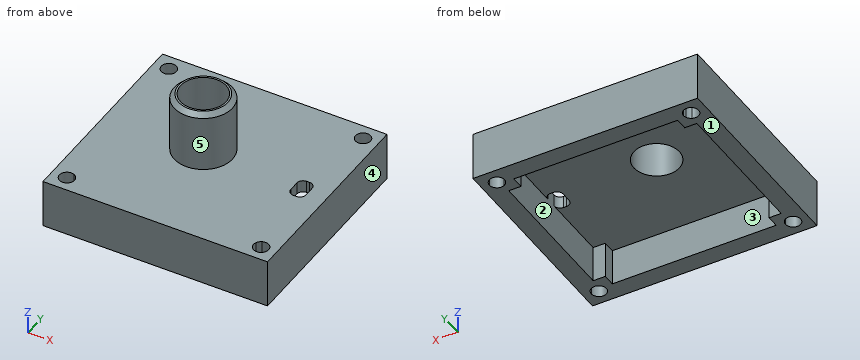
from build123d import *

# Parameters (mm, degrees)
F0_W     = 37
F0_H     = 34
F1_DEPTH = 8
F2_START = 6
F0_R     = 4.8
F2_DEPTH = 2
F3_R     = 1
F4_START = 6
F0_R_2   = 3.75
F4_DEPTH = 12
F5_SIZE  = 0.75


with BuildPart() as f1:
    # F0 (on Top) → F1 (new body)
    with BuildSketch(Plane.XY):
        with Locations((2.5, -1)):
            Rectangle(F0_W, F0_H)
        with BuildLine():
            Line((-12.3543560763, 13), (-11, 13))
            Line((-11, 13), (16, 13))
            Line((16, 13), (17.3543560763, 13))
            ThreePointArc((17.3543560763, 13), (18.2446129454, 14.7236328912), (19.75, 13.5))
            ThreePointArc((19.75, 13.5), (19.1846531969, 12.4541749668), (18, 12.3543560763))
            Line((18, 12.3543560763), (18, 11))
            Line((18, 11), (18, 0.875))
            Line((18, 0.875), (18, -2.875))
            Line((18, -2.875), (18, -13))
            Line((18, -13), (18, -14.3543560763))
            ThreePointArc((18, -14.3543560763), (19.1846531969, -14.4541749668), (19.75, -15.5))
            ThreePointArc((19.75, -15.5), (18.2446129454, -16.7236328912), (17.3543560763, -15))
            Line((17.3543560763, -15), (16, -15))
            Line((16, -15), (-11, -15))
            Line((-11, -15), (-12.3543560763, -15))
            ThreePointArc((-12.3543560763, -15), (-12.2763671088, -15.2446129454), (-12.25, -15.5))
            ThreePointArc((-12.25, -15.5), (-14.5458250332, -16.1846531969), (-13, -14.3543560763))
            Line((-13, -14.3543560763), (-13, -13))
            Line((-13, -13), (-13, 11))
            Line((-13, 11), (-13, 12.3543560763))
            ThreePointArc((-13, 12.3543560763), (-14.5458250332, 14.1846531969), (-12.25, 13.5))
            ThreePointArc((-12.25, 13.5), (-12.2763671088, 13.2446129454), (-12.3543560763, 13))
        make_face(mode=Mode.SUBTRACT)
        with BuildLine():
            Line((-11, -13), (-13, -13))
            Line((-13, -13), (-13, -14.3543560763))
            ThreePointArc((-13, -14.3543560763), (-12.6161165235, -14.6161165235), (-12.3543560763, -15))
            Line((-12.3543560763, -15), (-11, -15))
            Line((-11, -15), (-11, -13))
        make_face()
        with BuildLine():
            Line((18, -14.3543560763), (18, -13))
            Line((18, -13), (16, -13))
            Line((16, -13), (16, -15))
            Line((16, -15), (17.3543560763, -15))
            ThreePointArc((17.3543560763, -15), (17.6161165235, -14.6161165235), (18, -14.3543560763))
        make_face()
        with BuildLine():
            Line((17.3543560763, 13), (16, 13))
            Line((16, 13), (16, 11))
            Line((16, 11), (18, 11))
            Line((18, 11), (18, 12.3543560763))
            ThreePointArc((18, 12.3543560763), (17.6161165235, 12.6161165235), (17.3543560763, 13))
        make_face()
        with BuildLine():
            Line((-11, 11), (-11, 13))
            Line((-11, 13), (-12.3543560763, 13))
            ThreePointArc((-12.3543560763, 13), (-12.6161165235, 12.6161165235), (-13, 12.3543560763))
            Line((-13, 12.3543560763), (-13, 11))
            Line((-13, 11), (-11, 11))
        make_face()
    extrude(amount=F1_DEPTH)

    # F0 (on Top) → F2 (join)
    with BuildSketch(Plane.XY.offset(F2_START)):
        Polygon((16, 13), (-11, 13), (-11, 11), (-13, 11), (-13, -13), (-11, -13), (-11, -15), (16, -15), (16, -13), (18, -13), (18, -2.875), (15.5, -2.875), (15.5, 0.875), (18, 0.875), (18, 11), (16, 11), align=None)
        Circle(F0_R, mode=Mode.SUBTRACT)
    extrude(amount=F2_DEPTH)

    # F3
    f3_edges = [f1.edges().sort_by_distance(p)[0] for p in [
        (15.5, 0.875, 7),
        (18, 0.875, 7),
        (15.5, -2.875, 7),
        (18, -2.875, 7),
    ]]
    fillet(f3_edges, radius=F3_R)

    # F0 (on Top) → F4 (join)
    with BuildSketch(Plane.XY.offset(F4_START)):
        Circle(F0_R)
        Circle(F0_R_2, mode=Mode.SUBTRACT)
    extrude(amount=F4_DEPTH)

    # F5
    f5_edges = [f1.edges().sort_by_distance(p)[0] for p in [
        (-4.8, 0, 18),
    ]]
    chamfer(f5_edges, length=F5_SIZE)


solid = f1.part
CAD build for the part. Positions are in the model's coordinates, mm. Face numbers are marked on the shaded views. A direction names the side the tool comes from. Coordinates: 2 decimals unless noted, no trailing zeros. Write each loop counter-clockwise with the first axis right and the second up, starting at its lowest first coordinate (ties: lowest second). Pieces come first, ordered by that corner, then holes. Notation, with made-up numbers: M 82,79.5 L 127,79.5 A8 cw 127,91.5 Z; hole C 60.5,84 d10. An arc over 180 degrees is marked long. Return JSON: item names as keys, results as strings.
Item 1: Two-plate mould, pull along X, no slides. Class the marked faces 3, 4 and 5: +X half, -X half, draft (parallel to the pull), parting line (faces both ways), or undercut.
Findings below:
{"face 3": "undercut", "face 4": "+X half", "face 5": "parting line"}
Item 2: Slice it at A-A, the plane x = 0. Write the cut outline in (y, z).
Findings below:
{"outline": "M -18,0 L -15,0 L -15,6 L -3.75,6 L -3.75,18 L -4.05,18 L -4.8,17.25 L -4.8,8 L -18,8 Z; M 3.75,6 L 13,6 L 13,0 L 16,0 L 16,8 L 4.8,8 L 4.8,17.25 L 4.05,18 L 3.75,18 Z"}
Item 3: Slice it at B-B, the plane y = 5.5. Write the cut outline in (x, z), and give its area (3 significant figures).
Findings below:
{"outline": "M -16,0 L -13,0 L -13,6 L 18,6 L 18,0 L 21,0 L 21,8 L -16,8 Z", "area": "110 mm2"}
Item 4: Which spindle directions (+Z, -Z, +X, -X, +Y, -Y) get a long thin tool onto all of the face, cutting with end or side? Do the marked faces 1 and 2. Say none if no direction does.
Findings below:
{"face 1": "-Z, +X, -X, +Y, -Y", "face 2": "-Z"}
Item 5: Drop flat-ended pins along their axis: pin 1 Ø5 at (x, y) = (3, -4.5) entering from -Z; pin 2 Ø4 at (x, y) = (-13.5, -15.5) entering from +Z. Give the stop position or say it passes through.
Findings below:
{"pin 1": "stops at z = 6", "pin 2": "stops at z = 8"}
Item 6: Probe line 1 (X direction, y = -15.5, z = 5.75); line 2 (Y direction, x = 18.5, z = 4.5); line 3 (Y direction, x = 0, z = 12.75). List the from-to ranges inside material, lowest first. Write a range as from..to.
Findings below:
{"line 1": "x = -16..-14.75, -12.25..17.25, 19.75..21", "line 2": "y = -18..-16.75, -14.25..12.25, 14.75..16", "line 3": "y = -4.8..-3.75, 3.75..4.8"}
Item 7: Slice it at C-C, the plane z = 2.25. Write the cut outline in (x, y).
Findings below:
{"outline": "M -16,-18 L 21,-18 L 21,16 L -16,16 Z; hole C -13.5,-15.5 d2.5; hole C -13.5,13.5 d2.5; hole M -13,-13 L -11,-13 L -11,-15 L 16,-15 L 16,-13 L 18,-13 L 18,11 L 16,11 L 16,13 L -11,13 L -11,11 L -13,11 Z; hole C 18.5,-15.5 d2.5; hole C 18.5,13.5 d2.5"}
Item 8: Slice it at D-D, the plane x = -13.5. Write the cut outline in (y, z), and give its area (3 significant figures).
Findings below:
{"outline": "M -18,0 L -16.75,0 L -16.75,8 L -18,8 Z; M -14.25,0 L 12.25,0 L 12.25,8 L -14.25,8 Z; M 14.75,0 L 16,0 L 16,8 L 14.75,8 Z", "area": "232 mm2"}
